Input: dimensioned drawing with shaded views. Units: mm. Origin: part minimum x, y, z. A direction names the side the tool comes from. Coordinates: 2 decimals unless noted, no trailing zeros. Loops run counter-clockwise (first coordinate to the right, second up) from the corner with the lowest first, then second, coordinate; pieces in that order, holes last. Notation, with made-up numbers: (84, -31) - (111, -31) arc R11 ccw to (111, -26) - close; hole circle Ø6 at (75, 88.25). An arc over 180 degrees is marked (long way). Put each result on its own line as item: value. Start each with the question number.
1) Section B-B on y = 10. Output: boundary loops of the cut face in (x, z).
2) Contact query for flat-ended pins moving along their axis: pin 1 Ø8 at (x, y) = (28, 11) entering from -Z; pin 2 Ø10 at (x, y) = (21.5, 6.5) entering from +Z. Output: stop coordinate, or through.
3) Section A-A on x = 42.5. Output: boundary loops of the cut face in (y, z), and give its area (3 significant figures).
4) Section C-C on y = 15.5. Output: boundary loops of the cut face in (x, z).
5) Section D-D on x = 10. Output: boundary loops of the cut face in (y, z).
6) Reachability of the marked faces 1 and 2 from +Z, -Z, +X, -X, +Y, -Y: full face, straight path, thin tool, end or side. Return the list, or none.
7) Material intervals for line 1 along Z through (x, y) = (7.5, 5.75); line 2 along X through (y, z) = (17.5, 2.2); line 3 along X through (y, z) = (1.5, 1.55), sorted ascending. Write a range as from..to.
8) Draft query along X for the marked faces 3, 4 and 5. Return one class per face: +X half, -X half, draft (parallel to the pull), parting line (faces both ways), or undercut.
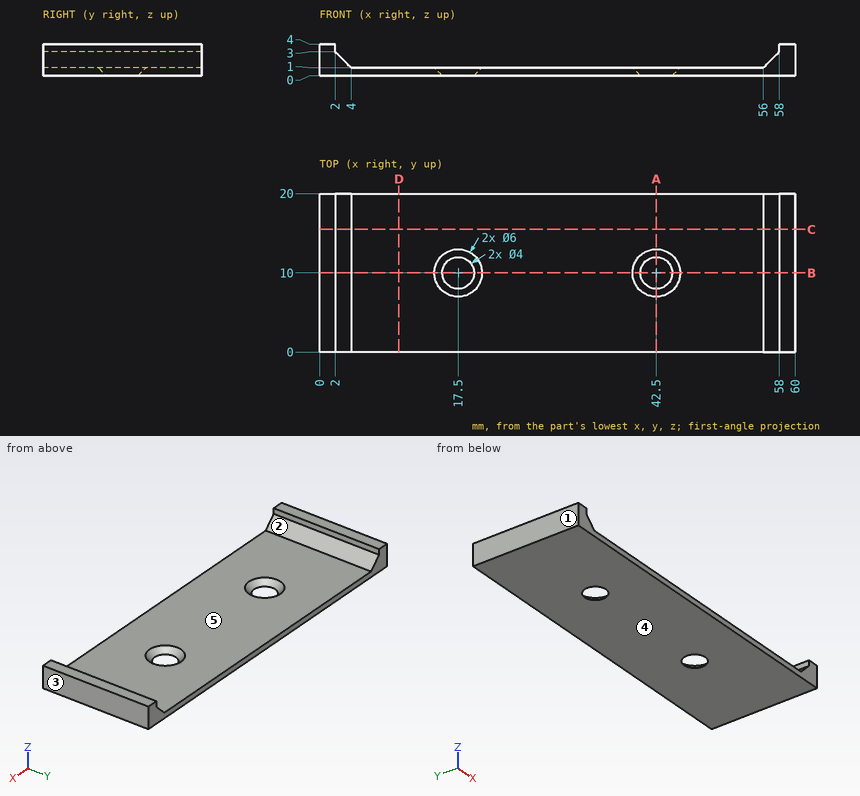
Answer block:
1. outline: (0, 0) - (15.5, 0) - (14.5, 1) - (4, 1) - (2, 3) - (2, 4) - (0, 4) - close; (19.5, 0) - (40.5, 0) - (39.5, 1) - (20.5, 1) - close; (44.5, 0) - (60, 0) - (60, 4) - (58, 4) - (58, 3) - (56, 1) - (45.5, 1) - close
2. pin 1: stops at z = 0
2. pin 2: stops at z = 1
3. outline: (0, 0) - (8, 0) - (7, 1) - (0, 1) - close; (12, 0) - (20, 0) - (20, 1) - (13, 1) - close
3. area: 15.0 mm²
4. outline: (0, 0) - (60, 0) - (60, 4) - (58, 4) - (58, 3) - (56, 1) - (4, 1) - (2, 3) - (2, 4) - (0, 4) - close
5. outline: (0, 0) - (20, 0) - (20, 1) - (0, 1) - close
6. face 1: +Z, -Z, -X, +Y, -Y
6. face 2: +Z, +Y, -Y
7. line 1: z = 0..1
7. line 2: x = 0..2.8, 57.2..60
7. line 3: x = 0..3.45, 56.55..60
8. face 3: +X half
8. face 4: draft
8. face 5: undercut
